```python
from build123d import *

# Parameters (mm, degrees)
SKETCH4_W               = 2.032
SKETCH4_H               = 2.54
SKETCH5_R               = 76.2
SKETCH5_R_2             = 31.75
BOSS_EXTRUDE1_DEPTH     = 3.81
SKETCH6_R               = 76.2
SKETCH6_R_2             = 62.23
BOSS_EXTRUDE2_DEPTH     = 10.16
CUT_EXTRUDE1_DEPTH      = 113.342968182
CUT_EXTRUDE1_DEPTH_BACK = 113.342968182
SKETCH2_R               = 6.35
SKETCH3_R               = 3.175
CUT_EXTRUDE2_DEPTH      = 113.342968182
CIRPATTERN1_COUNT       = 8


with BuildPart() as part:
    # Sketch1 → Revolve1 (revolve)
    with BuildSketch(Plane.XY, mode=Mode.PRIVATE) as revolve1_sk:
        with BuildLine():
            Line((0, 76.2), (-10.16, 76.2))
            Line((-10.16, 76.2), (-10.16, 21.082))
            ThreePointArc((-10.16, 21.082), (-11.647897552, 17.489897552), (-15.24, 16.002))
            Line((-15.24, 16.002), (-31.75, 16.002))
            Line((-31.75, 16.002), (-31.75, 9.652))
            Line((-31.75, 9.652), (-6.35, 9.652))
            Line((-6.35, 9.652), (-6.35, 19.812))
            ThreePointArc((-6.35, 19.812), (-5.606051224, 21.608051224), (-3.81, 22.352))
            Line((-3.81, 22.352), (0, 22.352))
            Line((0, 22.352), (0, 76.2))
        make_face()
    revolve(revolve1_sk.sketch.rotate(Axis((0, 0, 0), (-1, 0, 0)), 90), axis=Axis((0, 0, 0), (-1, 0, 0)))

    # Sketch4 → Cut-Revolve1 (revolve, cut)
    with BuildSketch(Plane.XY):
        with Locations((-1.016, 24.892)):
            Rectangle(SKETCH4_W, SKETCH4_H)
    revolve(axis=Axis((0, 0, 0), (-1, 0, 0)), mode=Mode.SUBTRACT)

    # Sketch5 → Boss-Extrude1 (add)
    with BuildSketch(Plane(origin=(0, 0, 0), x_dir=(0, 0, -1), z_dir=(1, 0, 0))):
        Circle(SKETCH5_R)
        with Locations(Location((0, 0, 0), (0, 0, 180))):
            Circle(SKETCH5_R_2, mode=Mode.SUBTRACT)
    extrude(amount=BOSS_EXTRUDE1_DEPTH)

    # Sketch6 → Boss-Extrude2 (add)
    with BuildSketch(Plane(origin=(3.81, 0, 0), x_dir=(0, 0, -1), z_dir=(1, 0, 0))):
        Circle(SKETCH6_R)
        Circle(SKETCH6_R_2, mode=Mode.SUBTRACT)
    extrude(amount=BOSS_EXTRUDE2_DEPTH)

    # Sketch2 → Cut-Extrude1 (cut, two sides: drawn at the far end of the back side and taken through both)
    with BuildSketch(Plane(origin=(0, 0, 0), x_dir=(0, 0, -1), z_dir=(1, 0, 0)).offset(-CUT_EXTRUDE1_DEPTH_BACK)):
        with Locations((41.275, 0)):
            Circle(SKETCH2_R)
        with Locations((-41.275, 0)):
            Circle(SKETCH2_R)
    extrude(amount=CUT_EXTRUDE1_DEPTH + CUT_EXTRUDE1_DEPTH_BACK, mode=Mode.SUBTRACT)

    # Sketch3 → Cut-Extrude2 (cut, symmetric)
    with BuildSketch(Plane(origin=(0, 0, 0), x_dir=(0, 0, -1), z_dir=(1, 0, 0))):
        with Locations((66.802, 0)):
            Circle(SKETCH3_R)
    cut_extrude2 = extrude(amount=CUT_EXTRUDE2_DEPTH, both=True, mode=Mode.SUBTRACT)

    # CirPattern1: Cut-Extrude2 ×8 about axis
    cirpattern1_axis = Axis((0, 0, 0), (1, 0, 0))
    for i in range(1, CIRPATTERN1_COUNT):
        add(cut_extrude2.rotate(cirpattern1_axis, i * 360 / CIRPATTERN1_COUNT), mode=Mode.SUBTRACT)


solid = part.part
```
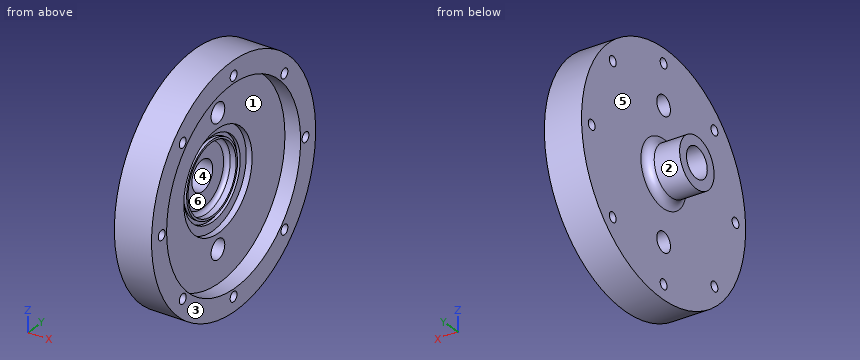
The model under review builds one solid part; all positions refer to its coordinate system, in mm. Face numbers are marked on the shaded views. A direction names the side the tool comes from. Give positions to 0.01 mm unless a question says otherwise; leave off trailing zeros. Write each loop counter-clockwise with the first axis right and the second up, starting at its lowest first coordinate (ties: lowest second). Pieces come first, ordered by that corner, then holes. Notation, with made-up numbers: M 50.25,-5.75 L 97.25,-5.75 A13 ccw 97.25,7.25 Z; hole C 76.25,58.25 d7. An arc over 180 degrees is marked long. Answer in a Markdown table with one row per item.
Item 1: Tool access review of the marked faces 4, 5 and 6: name each direction out of +Z, -Z, +X, -X, +Y, -Y from which nothing blocks a thin tool from reaching the whole face with its end or side.
Check sheet entries:
| item | result |
|---|---|
| face 4 | +X, -X |
| face 5 | -X |
| face 6 | +X |
Item 2: Add section D-D on y = 40. Give the boundary of the cut face in (x, z).
Check sheet entries:
| item | result |
|---|---|
| outline | M -10.16,-64.86 L 13.97,-64.86 L 13.97,-47.67 L 3.81,-47.67 L 3.81,47.67 L 13.97,47.67 L 13.97,64.86 L -10.16,64.86 Z |
Item 3: For line 1 along Z through (x, y) = (-5.5, -49.5); line 2 along Z through (x, y) = (-4.5, -5); line 3 along Y through (x, z) = (0, -46), list the stretches that pass through material, from the lowest coordinate up.
Check sheet entries:
| item | result |
|---|---|
| line 1 | -57.93 to -49.46, -45.01 to 45.01, 49.46 to 57.93 |
| line 2 | -76.04 to -45.19, -37.36 to -21.69, 21.69 to 37.36, 45.19 to 76.04 |
| line 3 | -60.75 to -50.16, -44.31 to -4.24, 4.24 to 44.31, 50.16 to 60.75 |
Item 4: For P1, Ø12, axis at y = 49, z = 27.5, coming from the +X side; P2, Ø23.5, axis at y = -0.5, z = -2, coming from the +X side; P3, Ø10, axis at y = 0, z = 66.802, coming from the -X side, all flat-tipped, find the tip position at first contact; note any pin that passes through.
Check sheet entries:
| item | result |
|---|---|
| P1 | x = 3.81 |
| P2 | x = -6.35 |
| P3 | x = -10.16 |
Item 5: Add section A-A on z = 0. State how many separate pieces and enclosed holes the cut face has, plus the area to 3 significant figures.
Check sheet entries:
| item | result |
|---|---|
| separate pieces | 4 |
| enclosed holes | 0 |
| area | 1,780 mm2 |
Item 6: Draft analysis for pull direction Y (two halves, no side actions). For the marked faces 1, 2 and 3, state which applies: +Y half, -Y half, draft (parallel to the pull), parting line (faces both ways), or undercut.
Check sheet entries:
| item | result |
|---|---|
| face 1 | undercut |
| face 2 | parting line |
| face 3 | draft |
Item 7: Add section B-B on x = -26. Give the boundary of the cut face in (y, z).
Check sheet entries:
| item | result |
|---|---|
| outline | C 0,0 d32; hole C 0,0 d19.3 |
